The listing builds one solid part. Answer for the finished solid, in the listing's coordinates (mm). A direction names the side the tool comes from. Give positions to 0.01 mm unless a question says otherwise; leave off trailing zeros. Order: outer loops, then holes, each group sorted by start corner. A loop starts at its lowest first (then second) coordinate and runs counter-clockwise, first axis right, second up.
```python
from build123d import *

# Parameters (mm, degrees)
SKETCH1_W                        = 38.1
SKETCH1_H                        = 12.7
BOSS_EXTRUDE1_DEPTH              = 250.825
SKETCH2_R                        = 6.35
CUT_EXTRUDE1_DEPTH               = 252.867769127
F_1_4_20_TAPPED_HOLE1_AT_2_COUNT = 2
F_1_4_20_TAPPED_HOLE1_AT_2_PITCH = 25.4
CHAMFER1_SIZE                    = 3.175
CUT_EXTRUDE2_DEPTH               = 9.525
CUT_EXTRUDE3_DEPTH               = 252.727647965


with BuildPart() as part:
    # Sketch1 → Boss-Extrude1 (new, symmetric)
    with BuildSketch(Plane(origin=(0, 0, 0), x_dir=(0, 0, -1), z_dir=(1, 0, 0))):
        Rectangle(SKETCH1_W, SKETCH1_H)
    extrude(amount=BOSS_EXTRUDE1_DEPTH, both=True)

    # Sketch2 → Cut-Extrude1 (cut, through all)
    with BuildSketch(Plane(origin=(0, 6.35, 0), x_dir=(1, 0, 0), z_dir=(0, 1, 0))):
        with Locations(Location((0, 0, 0), (0, 0, 270))):
            Circle(SKETCH2_R)
    extrude(amount=-CUT_EXTRUDE1_DEPTH, mode=Mode.SUBTRACT)

    # Sketch3 → 1/4-20 Tapped Hole1 (revolve, cut)
    with BuildSketch(Plane(origin=(250.825, 0, 12.7), x_dir=(0, 0, -1), z_dir=(0, 1, 0))):
        Polygon((0, 0), (0, 30.743816902), (2.5527, 29.21), (2.5527, 0), align=None)
    f_1_4_20_tapped_hole1 = revolve(axis=Axis((257.175, 0, 12.7), (-1, 0, 0)), mode=Mode.SUBTRACT)

    # 1/4-20 Tapped Hole1 at 2: 1/4-20 Tapped Hole1 ×2
    with Locations(*[(0, 0, -i * F_1_4_20_TAPPED_HOLE1_AT_2_PITCH) for i in range(1, F_1_4_20_TAPPED_HOLE1_AT_2_COUNT)]):
        add(f_1_4_20_tapped_hole1, mode=Mode.SUBTRACT)

    # Chamfer1
    chamfer1_edges = [part.edges().sort_by_distance(p)[0] for p in [
        (-250.825, 6.35, 0),
        (250.825, 6.35, 0),
    ]]
    chamfer(chamfer1_edges, length=CHAMFER1_SIZE)

    # Sketch4 → Cut-Extrude2 (cut)
    with BuildSketch(Plane.XZ.offset(6.35)):
        with BuildLine():
            Line((-215.9, -12.7), (-12.7, -12.7))
            ThreePointArc((-12.7, -12.7), (-9.860193669, -10.944903166), (-10.16, -7.62))
            ThreePointArc((-10.16, -7.62), (-12.7, 0), (-10.16, 7.62))
            ThreePointArc((-10.16, 7.62), (-9.860193669, 10.944903166), (-12.7, 12.7))
            Line((-12.7, 12.7), (-215.9, 12.7))
            ThreePointArc((-215.9, 12.7), (-218.14506403, 11.77006403), (-219.075, 9.525))
            Line((-219.075, 9.525), (-219.075, -9.525))
            ThreePointArc((-219.075, -9.525), (-218.14506403, -11.77006403), (-215.9, -12.7))
        make_face()
        with BuildLine():
            Line((219.075, -9.525), (219.075, 9.525))
            ThreePointArc((219.075, 9.525), (218.14506403, 11.77006403), (215.9, 12.7))
            Line((215.9, 12.7), (12.7, 12.7))
            ThreePointArc((12.7, 12.7), (9.860193669, 10.944903166), (10.16, 7.62))
            ThreePointArc((10.16, 7.62), (12.7, 0), (10.16, -7.62))
            ThreePointArc((10.16, -7.62), (9.860193669, -10.944903166), (12.7, -12.7))
            Line((12.7, -12.7), (215.9, -12.7))
            ThreePointArc((215.9, -12.7), (218.14506403, -11.77006403), (219.075, -9.525))
        make_face()
    extrude(amount=-CUT_EXTRUDE2_DEPTH, mode=Mode.SUBTRACT)

    # Sketch5 → Cut-Extrude3 (cut, through all)
    with BuildSketch(Plane.XZ.offset(-3.175)):
        with BuildLine():
            Line((-212.725, 6.35), (-212.725, -6.35))
            ThreePointArc((-212.725, -6.35), (-210.951786793, -9.198792514), (-207.612799189, -8.865527383))
            Line((-207.612799189, -8.865527383), (-191.121376316, 3.834472617))
            ThreePointArc((-191.121376316, 3.834472617), (-190.052963676, 7.373187558), (-193.058577128, 9.525))
            Line((-193.058577128, 9.525), (-209.55, 9.525))
            ThreePointArc((-209.55, 9.525), (-211.79506403, 8.59506403), (-212.725, 6.35))
        make_face()
        with BuildLine():
            Line((-190.672373684, -3.834472617), (-174.180950811, 8.865527383))
            ThreePointArc((-174.180950811, 8.865527383), (-170.841963207, 9.198792514), (-169.06875, 6.35))
            Line((-169.06875, 6.35), (-169.06875, -6.35))
            ThreePointArc((-169.06875, -6.35), (-169.99868597, -8.59506403), (-172.24375, -9.525))
            Line((-172.24375, -9.525), (-188.735172872, -9.525))
            ThreePointArc((-188.735172872, -9.525), (-191.740786324, -7.373187558), (-190.672373684, -3.834472617))
        make_face()
        with BuildLine():
            Line((-119.0625, 6.35), (-119.0625, -6.35))
            ThreePointArc((-119.0625, -6.35), (-119.99243597, -8.59506403), (-122.2375, -9.525))
            Line((-122.2375, -9.525), (-138.728922872, -9.525))
            ThreePointArc((-138.728922872, -9.525), (-141.734536324, -7.373187558), (-140.666123684, -3.834472617))
            Line((-140.666123684, -3.834472617), (-124.174700811, 8.865527383))
            ThreePointArc((-124.174700811, 8.865527383), (-120.835713207, 9.198792514), (-119.0625, 6.35))
        make_face()
        with BuildLine():
            Line((-143.052327128, 9.525), (-159.54375, 9.525))
            ThreePointArc((-159.54375, 9.525), (-161.78881403, 8.59506403), (-162.71875, 6.35))
            Line((-162.71875, 6.35), (-162.71875, -6.35))
            ThreePointArc((-162.71875, -6.35), (-160.945536793, -9.198792514), (-157.606549189, -8.865527383))
            Line((-157.606549189, -8.865527383), (-141.115126316, 3.834472617))
            ThreePointArc((-141.115126316, 3.834472617), (-140.046713676, 7.373187558), (-143.052327128, 9.525))
        make_face()
        with BuildLine():
            Line((-69.05625, 6.35), (-69.05625, -6.35))
            ThreePointArc((-69.05625, -6.35), (-69.98618597, -8.59506403), (-72.23125, -9.525))
            Line((-72.23125, -9.525), (-88.722672872, -9.525))
            ThreePointArc((-88.722672872, -9.525), (-91.728286324, -7.373187558), (-90.659873684, -3.834472617))
            Line((-90.659873684, -3.834472617), (-74.168450811, 8.865527383))
            ThreePointArc((-74.168450811, 8.865527383), (-70.829463207, 9.198792514), (-69.05625, 6.35))
        make_face()
        with BuildLine():
            Line((-93.046077128, 9.525), (-109.5375, 9.525))
            ThreePointArc((-109.5375, 9.525), (-111.78256403, 8.59506403), (-112.7125, 6.35))
            Line((-112.7125, 6.35), (-112.7125, -6.35))
            ThreePointArc((-112.7125, -6.35), (-110.939286793, -9.198792514), (-107.600299189, -8.865527383))
            Line((-107.600299189, -8.865527383), (-91.108876316, 3.834472617))
            ThreePointArc((-91.108876316, 3.834472617), (-90.040463676, 7.373187558), (-93.046077128, 9.525))
        make_face()
        with BuildLine():
            Line((-19.05, 6.35), (-19.05, -6.35))
            ThreePointArc((-19.05, -6.35), (-19.97993597, -8.59506403), (-22.225, -9.525))
            Line((-22.225, -9.525), (-38.716422872, -9.525))
            ThreePointArc((-38.716422872, -9.525), (-41.722036324, -7.373187558), (-40.653623684, -3.834472617))
            Line((-40.653623684, -3.834472617), (-24.162200811, 8.865527383))
            ThreePointArc((-24.162200811, 8.865527383), (-20.823213207, 9.198792514), (-19.05, 6.35))
        make_face()
        with BuildLine():
            Line((-43.039827128, 9.525), (-59.53125, 9.525))
            ThreePointArc((-59.53125, 9.525), (-61.77631403, 8.59506403), (-62.70625, 6.35))
            Line((-62.70625, 6.35), (-62.70625, -6.35))
            ThreePointArc((-62.70625, -6.35), (-60.933036793, -9.198792514), (-57.594049189, -8.865527383))
            Line((-57.594049189, -8.865527383), (-41.102626316, 3.834472617))
            ThreePointArc((-41.102626316, 3.834472617), (-40.034213676, 7.373187558), (-43.039827128, 9.525))
        make_face()
    cut_extrude3 = extrude(amount=-CUT_EXTRUDE3_DEPTH, mode=Mode.SUBTRACT)

    # Mirror1: 1/4-20 Tapped Hole1, Cut-Extrude3 across plane
    add(f_1_4_20_tapped_hole1.mirror(Plane(origin=(0, 0, 0), x_dir=(0, 0, 1), z_dir=(1, 0, 0))), mode=Mode.SUBTRACT)
    add(cut_extrude3.mirror(Plane(origin=(0, 0, 0), x_dir=(0, 0, 1), z_dir=(1, 0, 0))), mode=Mode.SUBTRACT)

    # Mirror1 copy 1 sketch → Mirror1 copy 1 (revolve, cut)
    with BuildSketch(Plane(origin=(-250.825, 0, -12.7), x_dir=(0, 0, -1), z_dir=(0, 1, 0))):
        Polygon((0, 0), (0, -30.743816902), (2.5527, -29.21), (2.5527, 0), align=None)
    revolve(axis=Axis((-257.175, 0, -12.7), (-1, 0, 0)), mode=Mode.SUBTRACT)


solid = part.part
```
1) A tool of negligible diameter and unlimited length cuts with its end or side. For faces 5 (the flat face through (113, -2, -12.7)), 6 (the flat face through (4, -6.35, 9)), 7 (the flat face through (99.47, 4.74, -2.604)), from which of +Z, -Z, +X, -X, +Y, -Y can it reach the whole face along a straight path? Write none if from no direction.
Geometry says:
face 5: -Y
face 6: +Z, -Z, +X, -X, -Y
face 7: +Y, -Y
2) Given P1, Ø1, axis at y = 4.5, z = -3, coming from the +X side; P2, Ø1.6, axis at y = 5.5, z = 1.5, coming from the +X side; P3, Ø12.5, axis at x = 87, z = 4, coming from the -Y side (3 decimals); P4, Ø7.5, axis at x = 0, z = 0, coming from the +Y side, each flat-ended and moving along its own axis, determine where each tip first touches the part or whether it passes through.
Geometry says:
P1: stops at x = 250
P2: stops at x = 249.3
P3: stops at y = 3.175
P4: passes through
3) Find section B-B (x = -50.5). Write down the section's boundary in (y, z) (3 decimals).
Geometry says:
outline: (-6.35, -19.05) - (6.35, -19.05) - (6.35, -3.402) - (3.175, -3.402) - (3.175, -12.7) - (-6.35, -12.7) - close; (-6.35, 12.7) - (3.175, 12.7) - (3.175, 9.525) - (6.35, 9.525) - (6.35, 19.05) - (-6.35, 19.05) - close
4) Find section A-A (x = 0). Write down the section's boundary in (y, z).
Geometry says:
outline: (-6.35, -19.05) - (6.35, -19.05) - (6.35, -6.35) - (-6.35, -6.35) - close; (-6.35, 6.35) - (6.35, 6.35) - (6.35, 19.05) - (-6.35, 19.05) - close
5) Straight lines are drawn through the part: probe 1 along X at (y, z) = (-3.5, -1) (3 decimals); probe 2 along Z at (x, y) = (-231.75, 0); probe 3 along X at (y, z) = (-1.25, 8.5) (3 decimals). For each, find the intervals that lie inside material, in ascending order.
Geometry says:
probe 1: x = -250.825 to -219.075, -12.661 to -6.271, 6.271 to 12.661, 219.075 to 250.825
probe 2: z = -19.05 to -15.25, -10.15 to 10.15, 15.25 to 19.05
probe 3: x = -250.825 to -219.075, -9.695 to 9.695, 219.075 to 250.825
6) For a pull along Z with two mould halves and no side action, classify faces 1 (the flat face through (4, 0, 19.05)), 2 (the flat face through (250.825, -2, 0)), 3 (the flat face through (149.476, 4.74, -2.604)), 4 (the flat face through (4, 0, -19.05)) as +Z half, -Z half, draft (parallel to the pull), parting line (faces both ways), or undercut.
Geometry says:
face 1: +Z half
face 2: draft
face 3: undercut
face 4: -Z half
